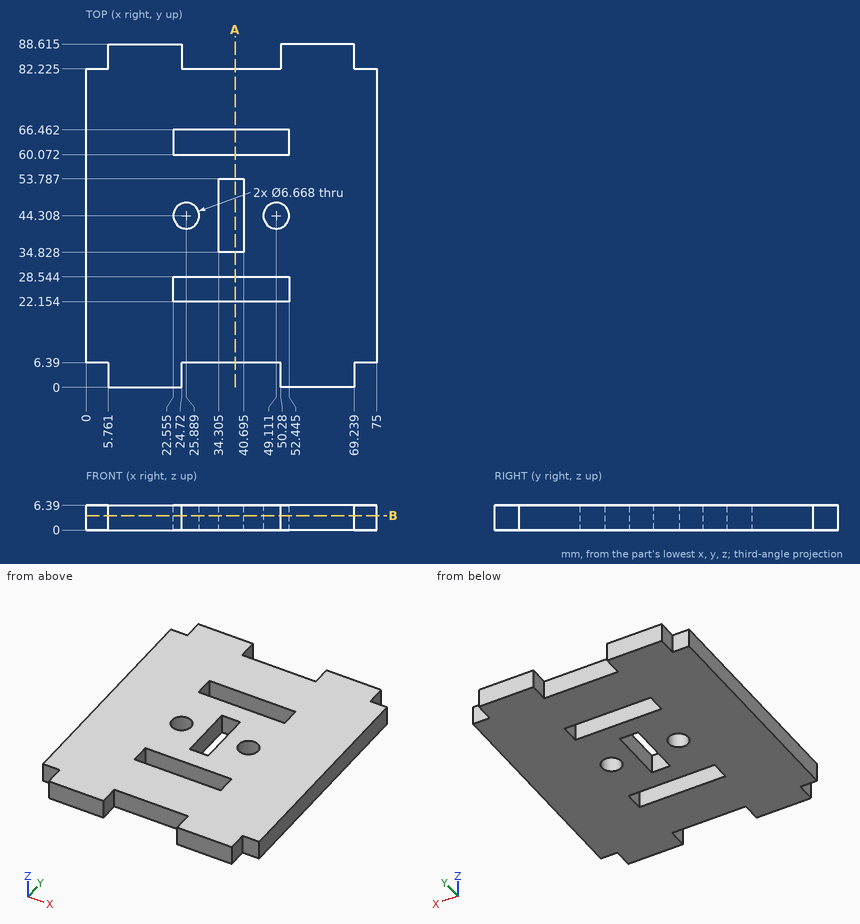
Part print with two shaded views. Sizes in mm from the minimum x, y, z corner. Round coordinates to 2 decimals unless told otherwise and drop trailing zeros. Order: outer loops, then holes, each group sorted by start corner. A loop starts at its lowest first (then second) coordinate and runs counter-clockwise, first axis right, second up. Notation, with made-up numbers: M -6,-1 L 38,-1 A19 ccw 38,19 Z; hole C 33.25,25 d11. An arc over 180 degrees is marked long. Answer in a Markdown table with one row per item. Add a question column.
Q1. Wall check: L1, parallel to Y at x = 41, z = 2 (1 decimal); L2, parallel to Y at x = 37, z = 4.5 (1 decimal); L3, parallel to X at y = 39.5, z = 0.75 (1 decimal). Give the ranges that are in metal, low to high. Write a range as from..to.
Q2. Pin check, flat tips, straight feed: pin 1 (3 mm diameter, centred on x = 32, z = 3, fed in from -Y); pin 2 (1.9 mm diameter, centred on y = 3, z = 3, fed in from -X); pin 3 (3 mm diameter, centred on x = 37, z = 2, fed in from +Y) (1 decimal). Stop position of each tip, or through.
Q3. Cut at A-A on x = 38.5. Give the cut face in (y, z) (1 decimal).
Q4. Cut at B-B on z = 3.75. Give the number of separate pieces and of enclosed holes in the cut face, and give its area (3 significant figures).
Established:
| question | item | result |
|---|---|---|
| 1 | L1 | y = 6.4..22.2, 28.5..60.1, 66.5..82.2 |
| 1 | L2 | y = 6.4..22.2, 28.5..34.8, 53.8..60.1, 66.5..82.2 |
| 1 | L3 | x = 0..34.3, 40.7..75 |
| 2 | pin 1 | stops at y = 6.39 |
| 2 | pin 2 | stops at x = 5.76 |
| 2 | pin 3 | stops at y = 82.2 |
| 3 | outline | M 6.4,0 L 22.2,0 L 22.2,6.4 L 6.4,6.4 Z; M 28.5,0 L 34.8,0 L 34.8,6.4 L 28.5,6.4 Z; M 53.8,0 L 60.1,0 L 60.1,6.4 L 53.8,6.4 Z; M 66.5,0 L 82.2,0 L 82.2,6.4 L 66.5,6.4 Z |
| 4 | separate pieces | 1 |
| 4 | enclosed holes | 5 |
| 4 | area | 5,600 mm2 |
